Design review of the part built by this model. Coordinates are the model's own, in mm. A direction names the side the tool comes from. Round coordinates to 2 decimals unless told otherwise and drop trailing zeros. Loops run counter-clockwise (first coordinate to the right, second up) from the corner with the lowest first, then second, coordinate; pieces in that order, holes last. Notation, with made-up numbers: (20.5, 14.5) - (56.5, 14.5) arc R14 cw to (56.5, 40.5) - close; hole circle Ø5 at (38.5, -10). An arc over 180 degrees is marked (long way). Return JSON: item names as keys, results as strings. Group by question number.
(1) For faces 1 (the flat face through (34.611, 31, 33)), 2 (the flat face through (-2, 31, 35.373)), 3 (the flat face through (19, 32.127, 64)), list the 3-axis set-ups (+Z, -Z, +X, -X, +Y, -Y) from which the entire face can be reached by the end or side of a thin tool; tool diameter is ignored.
(2) Clearance check with flat-ended pins moving along their axes: pin 1 (0.8 mm diameter, centred on x = 40.5, y = 31.5, fed in from -Z); pin 2 (0.8 mm diameter, centred on y = 31.5, z = 32, fed in from -X); pin 3 (0.8 mm diameter, centred on y = 31.5, z = 32.5, fed in from +X). State where each tip first meets the part, or that it passes through.
(3) We need section A-A, the plane y = 31.15. Write out the cut boundary in (x, z), and give its area (3 significant figures).
(4) We need section C-C, the plane x = 10. Write out the cut boundary in (y, z), and give its area (3 significant figures).
(5) We need section B-B, the plane z = 34. Write out the cut boundary in (x, y).
(6) Wall thickness on L1, parallel to X at y = 31.75, z = 32; L2, parallel to Z at x = -3, y = 31.25; L3, parallel to Z at x = 10, y = 30.95: over which ranges is each line inside the solid? List them lowest first. Write a range as [from, to].
from build123d import *

# Parameters (mm, degrees)
BOSS_EXTRUDE2_DEPTH = 1.5875


with BuildPart() as part:
    # Sketch3 → Boss-Extrude2 (new body)
    with BuildSketch(Plane(origin=(0, 30.53923904, 0), x_dir=(1, 0, 0), z_dir=(0, 1, 0))):
        with BuildLine():
            Line((46.80302417, -93.183255051), (46.80302417, -40.04646156))
            ThreePointArc((46.80302417, -40.04646156), (46.731182121, -40.016703609), (46.70142417, -39.94486156))
            ThreePointArc((46.70142417, -39.94486156), (46.731182121, -39.873019511), (46.80302417, -39.84326156))
            Line((46.80302417, -39.84326156), (46.80302417, -35.47446156))
            Line((46.80302417, -35.47446156), (46.80302417, -35.37286156))
            Line((46.80302417, -35.37286156), (46.70142417, -35.37286156))
            Line((46.70142417, -35.37286156), (34.71262417, -35.37286156))
            ThreePointArc((34.71262417, -35.37286156), (34.682866219, -35.444703609), (34.61102417, -35.47446156))
            ThreePointArc((34.61102417, -35.47446156), (34.539182121, -35.444703609), (34.50942417, -35.37286156))
            ThreePointArc((34.50942417, -35.37286156), (34.539182121, -35.301019511), (34.61102417, -35.27126156))
            Line((34.61102417, -35.27126156), (34.61102417, -29.88558893))
            ThreePointArc((34.61102417, -29.88558893), (34.539486295, -29.856142778), (34.50942417, -29.78486156))
            ThreePointArc((34.50942417, -29.78486156), (34.538144807, -29.713208308), (34.608937785, -29.682428156))
            ThreePointArc((34.608937785, -29.682428156), (19.371024177, -15.05286156), (4.637638035, -30.190416274))
            ThreePointArc((4.637638035, -30.190416274), (4.710051866, -30.219375736), (4.74059877, -30.29113436))
            ThreePointArc((4.74059877, -30.29113436), (4.711156288, -30.363523135), (4.63902417, -30.39358893))
            Line((4.63902417, -30.39358893), (4.63902417, -35.27126156))
            ThreePointArc((4.63902417, -35.27126156), (4.710866219, -35.301019511), (4.74062417, -35.37286156))
            ThreePointArc((4.74062417, -35.37286156), (4.710866219, -35.444703609), (4.63902417, -35.47446156))
            ThreePointArc((4.63902417, -35.47446156), (4.567182121, -35.444703609), (4.53742417, -35.37286156))
            Line((4.53742417, -35.37286156), (-8.46737583, -35.37286156))
            Line((-8.46737583, -35.37286156), (-8.56897583, -35.37286156))
            Line((-8.56897583, -35.37286156), (-8.56897583, -35.47446156))
            Line((-8.56897583, -35.47446156), (-8.56897583, -40.35126156))
            ThreePointArc((-8.56897583, -40.35126156), (-8.497133781, -40.381019511), (-8.46737583, -40.45286156))
            ThreePointArc((-8.46737583, -40.45286156), (-8.497133781, -40.524703609), (-8.56897583, -40.55446156))
            Line((-8.56897583, -40.55446156), (-8.56897583, -94.199276903))
            Line((-8.56897583, -94.199276903), (-8.56897583, -94.30086156))
            Line((-8.56897583, -94.30086156), (-8.497133781, -94.372703609))
            Line((-8.497133781, -94.372703609), (-7.116817879, -95.753019511))
            Line((-7.116817879, -95.753019511), (-7.04497583, -95.82486156))
            Line((-7.04497583, -95.82486156), (-6.943391173, -95.82486156))
            Line((-6.943391173, -95.82486156), (-5.11457583, -95.82486156))
            ThreePointArc((-5.11457583, -95.82486156), (-5.084817879, -95.753019511), (-5.01297583, -95.72326156))
            ThreePointArc((-5.01297583, -95.72326156), (-4.941133781, -95.753019511), (-4.91137583, -95.82486156))
            Line((-4.91137583, -95.82486156), (1.94703057, -95.82486156))
            Line((1.94703057, -95.82486156), (13.98703057, -95.82486156))
            Line((13.98703057, -95.82486156), (43.653417661, -95.82486156))
            Line((43.653417661, -95.82486156), (43.75502417, -95.82486156))
            Line((43.75502417, -95.82486156), (43.833075452, -95.759818825))
            Line((43.833075452, -95.759818825), (46.724972888, -93.349904295))
            Line((46.724972888, -93.349904295), (46.80302417, -93.28486156))
            Line((46.80302417, -93.28486156), (46.80302417, -93.183255051))
        make_face()
        with BuildLine():
            ThreePointArc((2.01053057, -93.28486156), (1.99193185, -93.329762841), (1.94703057, -93.34836156))
            ThreePointArc((1.94703057, -93.34836156), (1.902129289, -93.329762841), (1.88353057, -93.28486156))
            ThreePointArc((1.88353057, -93.28486156), (1.902129289, -93.239960279), (1.94703057, -93.22136156))
            ThreePointArc((1.94703057, -93.22136156), (1.99193185, -93.239960279), (2.01053057, -93.28486156))
        make_face(mode=Mode.SUBTRACT)
        with BuildLine():
            ThreePointArc((14.21053157, -93.28486156), (14.19193285, -93.329762841), (14.14703157, -93.34836156))
            ThreePointArc((14.14703157, -93.34836156), (14.102130289, -93.329762841), (14.08353157, -93.28486156))
            ThreePointArc((14.08353157, -93.28486156), (14.102130289, -93.239960279), (14.14703157, -93.22136156))
            ThreePointArc((14.14703157, -93.22136156), (14.19193285, -93.239960279), (14.21053157, -93.28486156))
        make_face(mode=Mode.SUBTRACT)
    extrude(amount=BOSS_EXTRUDE2_DEPTH)


solid = part.part
Solutions:
{
 "1": {"face 1": "-Z, +X, +Y, -Y", "face 2": "-Z, -X, +Y, -Y", "face 3": "+Z, -Z, +X, -X, +Y"},
 "2": {"pin 1": "z = 35.37", "pin 2": "x = 4.64", "pin 3": "x = 34.61"},
 "3": {"outline": "(-8.57, 35.37) - (4.54, 35.37) arc R0.1 cw (long way) to (4.64, 35.27) - (4.64, 30.39) arc R0.1 cw (long way) to (4.64, 30.19) arc R14.99 ccw to (34.61, 29.68) arc R0.1 cw to (34.61, 29.89) - (34.61, 35.27) arc R0.1 cw (long way) to (34.71, 35.37) - (46.8, 35.37) - (46.8, 39.84) arc R0.1 cw to (46.8, 40.05) - (46.8, 93.28) - (43.76, 95.82) - (-4.91, 95.82) arc R0.1 cw to (-5.11, 95.82) - (-7.04, 95.82) - (-8.57, 94.3) - (-8.57, 40.55) arc R0.1 cw to (-8.57, 40.35) - close; hole circle Ø0.13 at (1.95, 93.28); hole circle Ø0.13 at (14.15, 93.28)", "area": "3,850 mm^2"},
 "4": {"outline": "(30.54, 18.55) - (32.13, 18.55) - (32.13, 95.82) - (30.54, 95.82) - close", "area": "123 mm^2"},
 "5": {"outline": "(4.64, 30.54) - (34.61, 30.54) - (34.61, 32.13) - (4.64, 32.13) - close"},
 "6": {"L1": "[4.64, 34.61]", "L2": "[35.37, 95.82]", "L3": "[18.55, 95.82]"}
}
